```python
from build123d import *

# Parameters (mm, degrees)
DOME2_FACE_RADIUS               = 3.1
DOME2_HEIGHT                    = 0.8
SKETCH6_R                       = 0.500000006
CUT_EXTRUDE2_DEPTH              = 1
SKETCH7_R                       = 0.75
CUT_EXTRUDE3_DEPTH              = 1
BOSS_EXTRUDE1_REACH             = 12.152
SKETCH9_R                       = 1
SKETCH9_R_2                     = 0.45
BOSS_EXTRUDE1_DIRECTION_2_DEPTH = 0.5
SCALE1_SCALE                    = 2


with BuildPart() as part:
    # Sketch2 → Revolve2 (revolve)
    with BuildSketch(Plane.XY):
        with BuildLine():
            Line((0, 0), (3.1, 0))
            add(Edge.make_bspline(
                [(0, -10.151978408), (2.177642547, -9.857333884), (3.515065362, -5.793498011), (3.1, 0)],
                knots=[0, 0, 0, 0, 1, 1, 1, 1], degree=3))
            Line((0, -10.151978408), (0, 0))
        make_face()
    revolve(axis=Axis((0, -10.151978408, 0), (0, 1, 0)))

    # Dome2: a dome of height H over a round flat face of radius A is a cap of a sphere of radius (A * A + H * H) / (2 * H)
    dome2_r = (DOME2_FACE_RADIUS * DOME2_FACE_RADIUS + DOME2_HEIGHT * DOME2_HEIGHT) / (2 * DOME2_HEIGHT)
    dome2_base = Plane((0, 0, 0), z_dir=(0, -1, 0))
    with Locations(dome2_base.offset(DOME2_HEIGHT - dome2_r)):
        dome2_ball = Sphere(dome2_r, mode=Mode.PRIVATE)
    add(split(dome2_ball, bisect_by=dome2_base, keep=Keep.TOP, mode=Mode.PRIVATE), mode=Mode.SUBTRACT)

    # Sketch6 → Cut-Extrude2 (cut, symmetric)
    with BuildSketch(Plane(origin=(3.16696636, 0, 0), x_dir=(0, 0, -1), z_dir=(1, 0, 0))):
        with Locations((0, -1.377313707)):
            Circle(SKETCH6_R)
    cut_extrude2 = extrude(amount=CUT_EXTRUDE2_DEPTH, both=True, mode=Mode.SUBTRACT)

    # Mirror1: Cut-Extrude2 across plane
    add(cut_extrude2.mirror(Plane(origin=(0, 0, 0), x_dir=(0, 0, 1), z_dir=(1, 0, 0))), mode=Mode.SUBTRACT)

    # Sketch7 → Cut-Extrude3 (cut)
    with BuildSketch(Plane(origin=(0, 0, 0), x_dir=(1, 0, 0), z_dir=(0, 1, 0))):
        Circle(SKETCH7_R)
    extrude(amount=-CUT_EXTRUDE3_DEPTH, mode=Mode.SUBTRACT)

    # Sketch9 → Boss-Extrude1 (add, up to next)
    with BuildSketch(Plane(origin=(0, -10.151978408, 0), x_dir=(1, 0, 0), z_dir=(0, 1, 0)), mode=Mode.PRIVATE) as boss_extrude1_sk1:
        Circle(SKETCH9_R)
        Circle(SKETCH9_R_2, mode=Mode.SUBTRACT)
    boss_extrude1_tool1 = extrude(boss_extrude1_sk1.sketch, amount=BOSS_EXTRUDE1_REACH, mode=Mode.PRIVATE) - part.part
    add(boss_extrude1_tool1.solids().sort_by_distance((-0.971716, -10.151978, 0))[0])

    # Sketch9 → Boss-Extrude1 direction 2 (add)
    with BuildSketch(Plane(origin=(0, -10.151978408, 0), x_dir=(1, 0, 0), z_dir=(0, 1, 0))):
        Circle(SKETCH9_R)
        Circle(SKETCH9_R_2, mode=Mode.SUBTRACT)
    extrude(amount=-BOSS_EXTRUDE1_DIRECTION_2_DEPTH)


with BuildPart() as part_1:
    # Scale1: scaled about (3.7e-08, -4.298834834, 9.2e-08)
    add(part.part.scale(SCALE1_SCALE).moved(Location((-3.7e-08, 4.298834834, -9.2e-08))))


solid = part_1.part
```
Source: CAD feature listing. Evaluate the final solid. Frame: model axes, mm. A direction names the side the tool comes from. Round coordinates to 2 decimals unless told otherwise and drop trailing zeros. Use a Markdown table: item, result. Add a question column.
1. Contact query for flat-ended pins moving along their axis: P1, Ø0.6, axis at y = 1.5, z = 0.5, coming from the -X side; P2, Ø2, axis at y = 2, z = 0, coming from the +X side; P3, Ø1.5, axis at y = -3.5, z = 3.5, coming from the +X side; P4, Ø2.5, axis at x = 0, z = 0, coming from the -Y side. Output: stop coordinate, or through.
2. Line query: line 1 (X direction, y = -16.4, z = 0); line 2 (Y direction, x = 4.5, z = -0.25). Output: solid intervals per line, ascending.
3. Reachability of faces 1 (the flat face through (-4.334, 2, 0)), 2 (the cylindrical face through (-1.5, 2.55, -0.07)), 3 (the cylindrical face through (5.36, 0.57, 0.22)) from +Z, -Z, +X, -X, +Y, -Y: full face, straight path, thin tool, end or side. Return the list, or none.
Reported:
| question | item | result |
|---|---|---|
| 1 | P1 | stops at x = -4.33 |
| 1 | P2 | stops at x = 6.3 |
| 1 | P3 | stops at x = 5.57 |
| 1 | P4 | stops at y = -17.01 |
| 2 | line 1 | x = -2 to -0.9, 0.9 to 2 |
| 2 | line 2 | y = -11.47 to 0.58, 2.51 to 3.52 |
| 3 | face 1 | -X |
| 3 | face 2 | +Y |
| 3 | face 3 | +X |
